Design review of the part built by this model. Coordinates are the model's own, in mm. A direction names the side the tool comes from. Give positions to 0.01 mm unless a question says otherwise; leave off trailing zeros. Write each loop counter-clockwise with the first axis right and the second up, starting at its lowest first coordinate (ties: lowest second). Pieces come first, ordered by that corner, then holes. Notation, with made-up numbers: (6, 83) -> (14, 83) arc R26 cw to (14, 117) -> close; hole circle Ø7 at (41.5, 6.25). An arc over 180 degrees is marked (long way). Return JSON: item names as keys, results as strings. Group by question number.
from build123d import *

# Parameters (mm, degrees)
SKETCH_W     = 80
SKETCH_H     = 80
SKETCH_R     = 5
SKETCH_R_2   = 10
SKETCH_R_3   = 20
SKETCH_W_2   = 28.426124
SKETCH_H_2   = 28.426124
PAD_DEPTH    = 1.5
CHAMFER_SIZE = 1
FILLET_R     = 6


with BuildPart() as part:
    # Sketch → Pad (new body)
    with BuildSketch(Plane.XY):
        with Locations((40, -40)):
            Rectangle(SKETCH_W, SKETCH_H)
        with Locations((22.808456, -33.825606)):
            Circle(SKETCH_R, mode=Mode.SUBTRACT)
        with Locations((15.587115, -14.692374)):
            Circle(SKETCH_R_2, mode=Mode.SUBTRACT)
        with Locations((53.731579, -23.05761)):
            Circle(SKETCH_R_3, mode=Mode.SUBTRACT)
        with BuildLine():
            Line((4.836625, -44.554906), (24.835676, -44.360099))
            ThreePointArc((23.667351, -63.288176), (34.416474, -54.451564), (24.835676, -44.360099))
            ThreePointArc((4.745591, -64.554699), (14.886633, -74.083006), (23.667351, -63.288176))
            Line((4.836625, -44.554906), (4.745591, -64.554699))
        make_face(mode=Mode.SUBTRACT)
        with Locations((56.404202, -60.349873)):
            Rectangle(SKETCH_W_2, SKETCH_H_2, mode=Mode.SUBTRACT)
    extrude(amount=PAD_DEPTH)

    # Chamfer
    chamfer_edges = [part.edges().sort_by_distance(p)[0] for p in [
        (42.19114, -60.349873, 1.5),
        (56.404202, -46.136811, 1.5),
        (70.617264, -60.349873, 1.5),
        (56.404202, -74.562935, 1.5),
        (4.791108, -54.554802, 1.5),
        (14.83615, -44.457503, 1.5),
        (14.886633, -74.083006, 1.5),
        (34.416474, -54.451564, 1.5),
        (33.731579, -23.05761, 1.5),
        (17.808456, -33.825606, 1.5),
        (5.587115, -14.692374, 1.5),
    ]]
    chamfer(chamfer_edges, length=CHAMFER_SIZE)

    # Fillet
    fillet_edges = [part.edges().sort_by_distance(p)[0] for p in [
        (80, 0, 0.75),
        (80, -80, 0.75),
        (0, -80, 0.75),
        (0, 0, 0.75),
    ]]
    fillet(fillet_edges, radius=FILLET_R)


solid = part.part
Q1. For L1, parallel to X at y = -38, z = 0.3; L2, parallel to Y at x = 9, z = 0.3; L3, parallel to Y at x = 22.5, z = 1.25, list the stretches that pass through material, from the lowest coordinate up. Write a range as from..to.
Q2. Insertion check: pin 1 (8 mm diameter, centred on x = 22.81, y = -33.83, fed in from -Z). The pin has a flat end and moves straight along its axis. Give the tip position at first contact, or say it passes through.
Q3. Mouldability with a two-part tool opening along X and no side actions: class faces 4 (the face through (1.711, -1.804, 0.76)), 5 (the face through (78.196, -78.289, 0.76)), 6 (the face through (33.75, -22.18, 0.25)) as +X half, -X half, draft (parallel to the pull), parting line (faces both ways), or undercut.
Q4. Take a section at B-B, the plane y = -13.5. Count the separate pieces of the cut face and the enclosed holes in it, plus the area to 3 significant figures.
Q5. Tool access review of faces 1 (the face through (34.4, -54.67, 0.25)), 2 (the face through (34.6, -54.24, 0.67)), 3 (the face through (39, -39, 0)): name each direction out of +Z, -Z, +X, -X, +Y, -Y from which nothing blocks a thin tool from reaching the whole face with its end or side.
Q6. Take a section at A-A, the plane z = 0.95. Give the boundary of the cut face in (x, y), plus the area to 3 significant figures.
Final values:
{
 "1": {"L1": "x = 0..20.06, 25.56..40.44, 67.03..80", "L2": "y = -80..-72.52, -44.51..-22.22, -7.17..0", "L3": "y = -80..-70.69, -43.63..-39.57, -28.08..-22.92, -6.46..0"},
 "2": {"pin 1": "passes through"},
 "3": {"face 4": "-X half", "face 5": "+X half", "face 6": "undercut"},
 "4": {"separate pieces": "3", "enclosed holes": "0", "area": "35.4 mm²"},
 "5": {"face 1": "+Z, -Z", "face 2": "+Z", "face 3": "-Z, +X, -X, +Y, -Y"},
 "6": {"outline": "(0, -74) arc R6 ccw to (6, -80) -> (74, -80) arc R6 ccw to (80, -74) -> (80, -6) arc R6 ccw to (74, 0) -> (6, 0) arc R6 ccw to (0, -6) -> close; hole (4.3, -64.55) arc R9.96 ccw (long way) to (24.18, -63.79) arc R9.96 ccw (long way) to (24.83, -43.91) -> (4.39, -44.11) -> close; hole circle Ø20.9 at (15.59, -14.69); hole circle Ø10.9 at (22.81, -33.83); hole circle Ø40.9 at (53.73, -23.06); hole (41.74, -75.01) -> (71.07, -75.01) -> (71.07, -45.69) -> (41.74, -45.69) -> close", "area": "3,020 mm²"}
}
